The listing builds one solid part. Answer for the finished solid, in the listing's coordinates (mm). Face numbers are marked on the shaded views. Round coordinates to 2 decimals unless told otherwise and drop trailing zeros. Write each loop counter-clockwise with the first axis right and the second up, starting at its lowest first coordinate (ties: lowest second). Pieces come first, ordered by that corner, then holes.
Item 1: Find the intervals of material crossed by probe 1 along Z at (x, y) = (2.5, 8.5); probe 2 along Z at (x, y) = (0.25, -9.5); probe 3 along Y at (x, z) = (1.35, -16), in increasing order.
Item 2: Find section D-D on y = 9. Give the vertices of the cut face in (x, z) (3 decimals).
Item 3: This flat-tipped pin is pushed along its axis until it touches: pin 1 (1 mm diameter, centred on x = 2, z = -8, fed in from -Y). Where does it stop, or does it pass through?
Item 4: Find section A-A on z = 0. Give the vertices of the cut face in (x, y) (1 decimal).
Item 5: Find section B-B on y = 0. Give the vertices of the cut face in (x, z) (1 decimal), then the cut area to 3 significant figures.
Item 6: For a pull along Z with two mould halves and no side action, classify the marked faces 1, 2 and 3 as +Z half, -Z half, draft (parallel to the pull), parting line (faces both ways), or undercut.
Item 7: Find section C-C on x = 0.85. Give the vertices of the cut face in (y, z) (1 decimal), then the cut area to 3 significant figures.
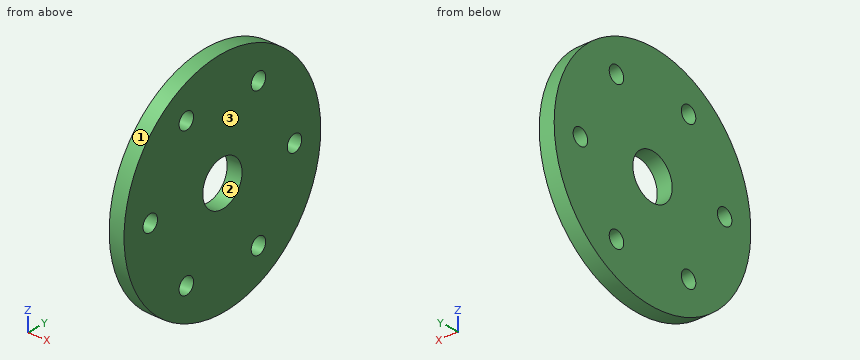
Autodesk Inventor part; units mm, degrees
ref_plane "YZ Plane" through (0, 0, 0) normal (1, 0, 0) x (0, 1, 0)
ref_plane "XZ Plane" through (0, 0, 0) normal (0, 1, 0) x (-1, 0, 0)
ref_plane "XY Plane" through (0, 0, 0) normal (0, 0, 1) x (1, 0, 0)
sketch "Sketch1" plane through (0, 0, 0) normal (1, 0, 0) x (0, 1, 0)
  circle A0 centre (0, 0) radius 23.8125
  circle A1 centre (0, 0) radius 17.4625 construction
  line L0 (0, 0) -> (23.8125, 0) construction
  circle A2 centre (17.4625, 0) radius 1.7526
  circle A3 centre (8.7313, 15.123) radius 1.7526
  circle A4 centre (-8.7312, 15.123) radius 1.7526
  circle A5 centre (-17.4625, 0) radius 1.7526
  circle A6 centre (-8.7313, -15.123) radius 1.7526
  circle A7 centre (8.7312, -15.123) radius 1.7526
  circle A8 centre (0, 0) radius 4.7625
  dimension "d0" = 47.625
  dimension "d1" = 34.925
  dimension "d2" = 3.5052
  dimension "d5" = 360
  dimension "d9" = 9.525
extrude "Extrusion1" add sketch "Sketch1" along normal blind 3.175
properties part number "Wheel Cover" material "UHMW, White"
Check values:
1. probe 1: z = -22.24 to -16.86, -13.39 to 13.39, 16.86 to 22.24
1. probe 2: z = -21.84 to -16.7, -13.55 to 13.55, 16.7 to 21.84
1. probe 3: y = -17.64 to -10.25, -7.21 to 7.21, 10.25 to 17.64
2. outline: (0, -22.046) - (3.175, -22.046) - (3.175, -16.855) - (0, -16.855) - close; (0, -13.391) - (3.175, -13.391) - (3.175, 13.391) - (0, 13.391) - close; (0, 16.855) - (3.175, 16.855) - (3.175, 22.046) - (0, 22.046) - close
3. pin 1: stops at y = -22.6
4. outline: (0, -23.8) - (3.2, -23.8) - (3.2, -19.2) - (0, -19.2) - close; (0, -15.7) - (3.2, -15.7) - (3.2, -4.8) - (0, -4.8) - close; (0, 4.8) - (3.2, 4.8) - (3.2, 15.7) - (0, 15.7) - close; (0, 19.2) - (3.2, 19.2) - (3.2, 23.8) - (0, 23.8) - close
5. outline: (0, -23.8) - (3.2, -23.8) - (3.2, -4.8) - (0, -4.8) - close; (0, 4.8) - (3.2, 4.8) - (3.2, 23.8) - (0, 23.8) - close
5. area: 121 mm2
6. face 1: parting line
6. face 2: undercut
6. face 3: draft
7. outline: circle Ø47.6 at (0, 0); hole circle Ø3.5 at (-17.5, 0); hole circle Ø3.5 at (-8.7, -15.1); hole circle Ø3.5 at (-8.7, 15.1); hole circle Ø9.5 at (0, 0); hole circle Ø3.5 at (8.7, -15.1); hole circle Ø3.5 at (8.7, 15.1); hole circle Ø3.5 at (17.5, 0)
7. area: 1,650 mm2
